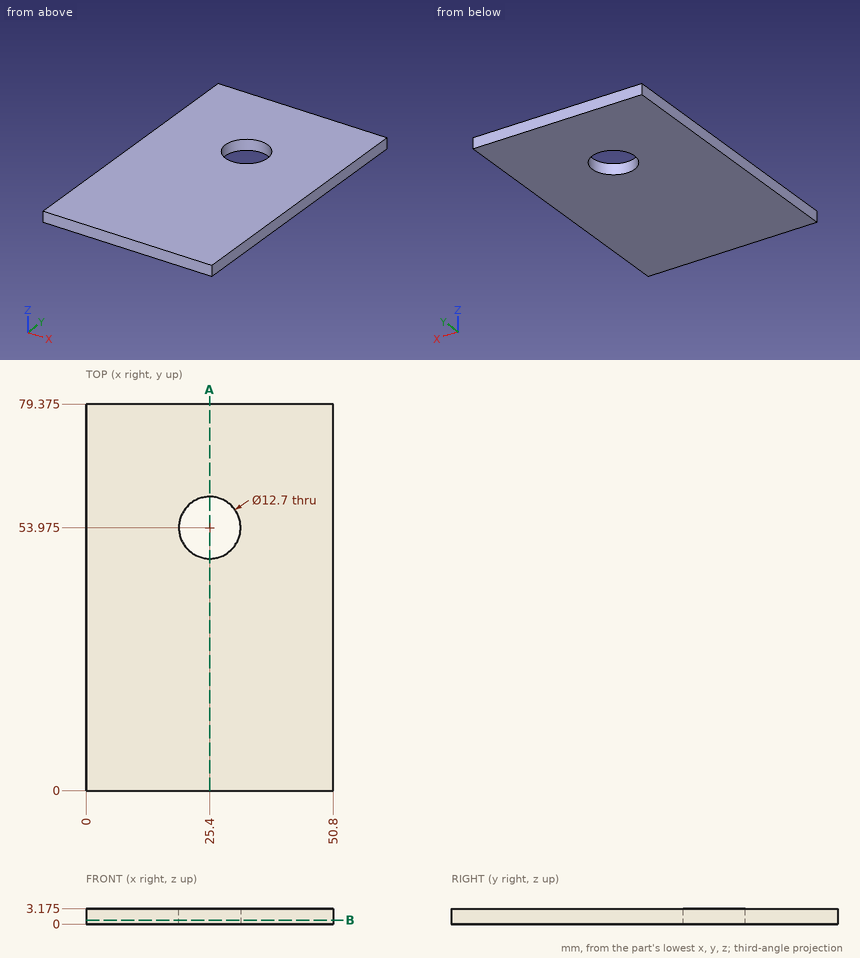
Print and shaded views of the part. All mm, measured from the part's lowest x, y and z. Give positions to 0.01 mm unless a question says otherwise; leave off trailing zeros. Loops run counter-clockwise (first coordinate to the right, second up) from the corner with the lowest first, then second, coordinate; pieces in that order, holes last. Notation, with made-up numbers: (-37.5, 12) - (-20.5, 12) arc R27 cw to (-20.5, 31) - close; hole circle Ø4 at (32.25, -25.5). An arc over 180 degrees is marked (long way). One line per item, written item: value. Start each with the question number.
1. Slice it at A-A (x = 25.4). List the corners of the cut face in (y, z) (3 decimals), plus the area to 3 significant figures.
2. Probe L1, parallel to Y at x = 25.4, z = 1.15 (3 decimals); L2, parallel to X at y = 58.5, z = 1.1; L3, parallel to Y at x = 26, z = 1.1 (3 decimals). List the from-to ranges inside material, lowest first. Write a range as from..to.
3. Slice it at B-B (z = 0.8). List the corners of the cut face in (x, y) (3 decimals).
Solution:
1. outline: (0, 0) - (47.625, 0) - (47.625, 3.175) - (0, 3.175) - close; (60.325, 0) - (79.375, 0) - (79.375, 3.175) - (60.325, 3.175) - close
1. area: 212 mm^2
2. L1: y = 0..47.625, 60.325..79.375
2. L2: x = 0..20.95, 29.85..50.8
2. L3: y = 0..47.653, 60.297..79.375
3. outline: (0, 0) - (50.8, 0) - (50.8, 79.375) - (0, 79.375) - close; hole circle Ø12.7 at (25.4, 53.975)
